Could you check a few things on this model? Use its own coordinates, in mm. Face numbers are marked on the shaded views. A direction names the side the tool comes from. Coordinates: 2 decimals unless noted, no trailing zeros. Loops run counter-clockwise (first coordinate to the right, second up) from the corner with the lowest first, then second, coordinate; pieces in that order, holes last. Notation, with made-up numbers: (70.25, -9.75) - (105.25, -9.75) arc R28 cw to (105.25, 28.25) - close; hole circle Ø4 at (2.5, 43). An arc over 180 degrees is marked (long way). Put each result on its own line as item: value. Start each with the question number.
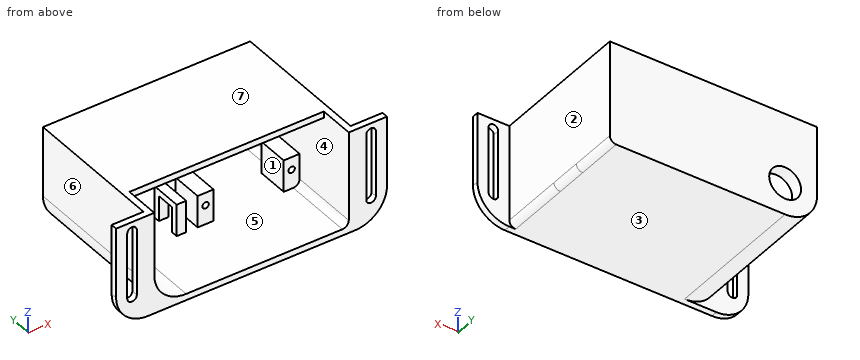
```python
from build123d import *

# Parameters (mm, degrees)
SKETCH2_W           = 85
SKETCH2_H           = 32
BOSS_EXTRUDE1_DEPTH = 2
SKETCH3_W           = 65
SKETCH3_H           = 32
BOSS_EXTRUDE2_DEPTH = 45
SKETCH4_W           = 61
SKETCH4_H           = 28
CUT_EXTRUDE1_DEPTH  = 43
FILLET1_R           = 10
FILLET2_R           = 2
FILLET3_R           = 10
FILLET4_R           = 10
FILLET5_R           = 10
FILLET6_R           = 2
SKETCH5_W           = 61
SKETCH5_H           = 22.301239178
CUT_EXTRUDE2_DEPTH  = 10
CUT_EXTRUDE3_DEPTH  = 10
SKETCH7_R           = 5
CUT_EXTRUDE4_DEPTH  = 10
SKETCH8_W           = 5
SKETCH8_H           = 12
SKETCH8_W_2         = 7
BOSS_EXTRUDE3_DEPTH = 10
FILLET8_R           = 2
SKETCH9_R           = 1
CUT_EXTRUDE5_DEPTH  = 10
SKETCH10_W          = 3
SKETCH10_H          = 10
BOSS_EXTRUDE4_DEPTH = 10
SKETCH11_W          = 8
SKETCH11_H          = 6
CUT_EXTRUDE6_DEPTH  = 5


with BuildPart() as part:
    # Sketch2 → Boss-Extrude1 (new body)
    with BuildSketch(Plane(origin=(0, 0, 0), x_dir=(1, 0, 0), z_dir=(0, 1, 0))):
        Rectangle(SKETCH2_W, SKETCH2_H)
    extrude(amount=BOSS_EXTRUDE1_DEPTH)

    # Sketch3 → Boss-Extrude2 (add)
    with BuildSketch(Plane(origin=(0, 2, 0), x_dir=(1, 0, 0), z_dir=(0, 1, 0))):
        Rectangle(SKETCH3_W, SKETCH3_H)
    extrude(amount=BOSS_EXTRUDE2_DEPTH)

    # Sketch4 → Cut-Extrude1 (cut)
    with BuildSketch(Plane.XZ):
        Rectangle(SKETCH4_W, SKETCH4_H)
    extrude(amount=-CUT_EXTRUDE1_DEPTH, mode=Mode.SUBTRACT)

    # Fillet1
    fillet1_edges = [part.edges().sort_by_distance(p)[0] for p in [
        (-32.5, 24.5, -16),
    ]]
    fillet(fillet1_edges, radius=FILLET1_R)

    # Fillet2
    fillet2_edges = [part.edges().sort_by_distance(p)[0] for p in [
        (32.5, 24.5, -16),
    ]]
    fillet(fillet2_edges, radius=FILLET2_R)

    # Fillet3
    fillet3_edges = [part.edges().sort_by_distance(p)[0] for p in [
        (-42.5, 1, -16),
    ]]
    fillet(fillet3_edges, radius=FILLET3_R)

    # Fillet4
    fillet4_edges = [part.edges().sort_by_distance(p)[0] for p in [
        (42.5, 1, -16),
    ]]
    fillet(fillet4_edges, radius=FILLET4_R)

    # Fillet5
    fillet5_edges = [part.edges().sort_by_distance(p)[0] for p in [
        (-30.5, 21.5, -14),
    ]]
    fillet(fillet5_edges, radius=FILLET5_R)

    # Fillet6
    fillet6_edges = [part.edges().sort_by_distance(p)[0] for p in [
        (30.5, 21.5, -14),
    ]]
    fillet(fillet6_edges, radius=FILLET6_R)

    # Sketch5 → Cut-Extrude2 (cut)
    with BuildSketch(Plane.XY.offset(16)):
        Rectangle(SKETCH5_W, SKETCH5_H)
    extrude(amount=-CUT_EXTRUDE2_DEPTH, mode=Mode.SUBTRACT)

    # Sketch6 → Cut-Extrude3 (cut)
    with BuildSketch(Plane(origin=(0, 2, 0), x_dir=(1, 0, 0), z_dir=(0, 1, 0))):
        with BuildLine():
            Line((39, 7.816649024), (39, -12.904408744))
            ThreePointArc((39, -12.904408744), (37.5, -14.404408744), (36, -12.904408744))
            Line((36, -12.904408744), (36, 7.816649024))
            ThreePointArc((36, 7.816649024), (37.5, 9.316649024), (39, 7.816649024))
        make_face()
        with BuildLine():
            Line((-36, 7.816649024), (-36, -12.904408744))
            ThreePointArc((-36, -12.904408744), (-37.5, -14.404408744), (-39, -12.904408744))
            Line((-39, -12.904408744), (-39, 7.816649024))
            ThreePointArc((-39, 7.816649024), (-37.5, 9.316649024), (-36, 7.816649024))
        make_face()
    extrude(amount=-CUT_EXTRUDE3_DEPTH, mode=Mode.SUBTRACT)

    # Sketch7 → Cut-Extrude4 (cut)
    with BuildSketch(Plane(origin=(0, 47, 0), x_dir=(1, 0, 0), z_dir=(0, 1, 0))):
        with Locations((-22.5, 6)):
            Circle(SKETCH7_R)
    extrude(amount=-CUT_EXTRUDE4_DEPTH, mode=Mode.SUBTRACT)

    # Sketch8 → Boss-Extrude3 (add)
    with BuildSketch(Plane(origin=(0, 22, 0), x_dir=(1, 0, 0), z_dir=(0, 1, 0))):
        with Locations((1, 10)):
            Rectangle(SKETCH8_W, SKETCH8_H)
        with Locations((29, 10)):
            Rectangle(SKETCH8_W_2, SKETCH8_H)
    extrude(amount=BOSS_EXTRUDE3_DEPTH)

    # Fillet8
    fillet8_edges = [part.edges().sort_by_distance(p)[0] for p in [
        (32.5, 27, -16),
    ]]
    fillet(fillet8_edges, radius=FILLET8_R)

    # Sketch9 → Cut-Extrude5 (cut)
    with BuildSketch(Plane.XZ.offset(-22)):
        with Locations((1, -8)):
            Circle(SKETCH9_R)
        with Locations((28, -8)):
            Circle(SKETCH9_R)
    extrude(amount=-CUT_EXTRUDE5_DEPTH, mode=Mode.SUBTRACT)

    # Sketch10 → Boss-Extrude4 (add)
    with BuildSketch(Plane.XY.offset(-14)):
        with Locations((-6.587930701, 27)):
            Rectangle(SKETCH10_W, SKETCH10_H)
    extrude(amount=BOSS_EXTRUDE4_DEPTH)

    # Sketch11 → Cut-Extrude6 (cut)
    with BuildSketch(Plane.ZY.offset(8.087930701)):
        with Locations((-10, 27)):
            Rectangle(SKETCH11_W, SKETCH11_H)
    extrude(amount=-CUT_EXTRUDE6_DEPTH, mode=Mode.SUBTRACT)


solid = part.part
```
(1) For pin 1 Ø3 at (y, z) = (31, 12) entering from +X; pin 2 Ø17.5 at (y, z) = (20, 9) entering from -X; pin 3 Ø0.9 at (x, z) = (-7, -10) entering from -Y, each with a flat end and sliding along its axis, tell me the tip position at first contact or that it passes through.
(2) I want a section at C-C on y = 14.5. List the corners of the cut face in (x, z) for me, and give its area (3 significant figures).
(3) I need wall thicknesses on L1, parallel to Y at x = 26, z = -8.5; L2, parallel to X at y = 45, z = -6; L3, parallel to Z at x = 1, y = 25. Which ranges of each line are inside material? Lowest first, please. Write a range as [from, to].
(4) I want a section at B-B on z = 11. List the corners of the cut face in (x, y) for me.
(5) Which directions (+Z, -Z, +X, -X, +Y, -Y) give clear straight access to the entire face, cutting with the end or side of a thin tool? Please do the marked faces 1, 2 and 3.
(6) If we mould it in two halves opening along X, with no side actions, what happens to the marked faces 4, 5, 6 and 7? For each: pulls with the +X half, pulls with the -X half, needs draft (parallel to the pull), parting line crosses it, or undercut.
(7) I want a section at A-A on x = 1. List the corners of the cut face in (y, z) for me.
(8) I want a section at D-D on x = 18. List the corners of the cut face in (y, z) for me.
Answer sheet:
1. pin 1: stops at x = 32.5
1. pin 2: stops at x = -32.5
1. pin 3: stops at y = 22
2. outline: (-32.5, -6) arc R10 ccw to (-22.5, -16) - (30.5, -16) arc R2 ccw to (32.5, -14) - (32.5, 16) - (-32.5, 16) - close; hole (-30.5, -4) arc R10 ccw to (-20.5, -14) - (28.5, -14) arc R2 ccw to (30.5, -12) - (30.5, 14) - (-30.5, 14) - close
2. area: 372 mm^2
3. L1: y = [22, 32], [43, 47]
3. L2: x = [-32.5, -27.5], [-17.5, 32.5]
3. L3: z = [-16, -9], [-7, -4], [14, 16]
4. outline: (-42.5, 0) - (-39, 0) - (-39, 2) - (-42.5, 2) - close; (-36, 0) - (-30.5, 0) - (-30.5, 43) - (30.5, 43) - (30.5, 0) - (36, 0) - (36, 2) - (32.5, 2) - (32.5, 47) - (-32.5, 47) - (-32.5, 2) - (-36, 2) - close; (39, 0) - (42.5, 0) - (42.5, 2) - (39, 2) - close
5. face 1: -Y
5. face 2: +Z, -Z, +X, +Y
5. face 3: -Z, +X, -X, +Y, -Y
6. face 4: undercut
6. face 5: undercut
6. face 6: pulls with the -X half
6. face 7: needs draft
7. outline: (0, -16) - (47, -16) - (47, 16) - (11.15, 16) - (11.15, 14) - (43, 14) - (43, -14) - (32, -14) - (32, -9) - (22, -9) - (22, -14) - (0, -14) - close; (22, -7) - (32, -7) - (32, -4) - (22, -4) - close
8. outline: (0, -16) - (47, -16) - (47, 16) - (11.15, 16) - (11.15, 14) - (43, 14) - (43, -14) - (0, -14) - close
